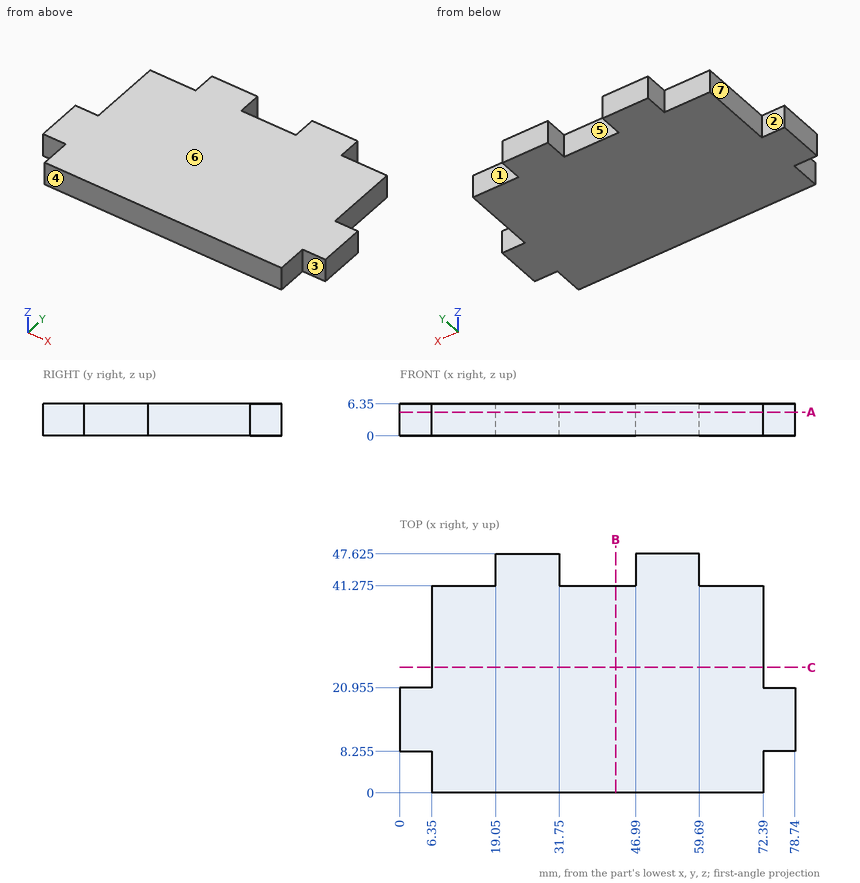
Here's the drawing with two shaded views (mm, measured from the low corner). I have some questions. A direction names the side the tool comes from. Coordinates: 2 decimals unless noted, no trailing zeros. Write each loop counter-clockwise with the first axis right and the second up, starting at its lowest first coordinate (ties: lowest second). Pieces come first, ordered by that corner, then holes.
Item 1: If I drill on line 1 (X direction, y = 43, z = 1.75); line 2 (X direction, y = 36, z = 6); line 3 (Y direction, x = 15, z = 5) (3 decimals), over which ranges is the centre line in solid material (lowest first)?
Item 2: I want a section at C-C on y = 25. Write out the boundary of the cut face in (x, z).
Item 3: I want a section at B-B on x = 43. Write out the boundary of the cut face in (y, z) (3 decimals).
Item 4: Will these pins go through, and if not, where does the flat tip stop? pin 1 (3 mm diameter, centred on x = 76, z = 2, fed in from +Y) (3 decimals); pin 2 (1.9 mm diameter, centred on x = 3.5, z = 3, fed in from -Y) (3 decimals); pin 3 (3 mm diameter, centred on x = 68.5, z = 3, fed in from +Y) (3 decimals).
Item 5: If we mould it in two halves opening along X, with no side actions, what happens to the marked faces 5, 6 and 7? For each: +X half, -X half, draft (parallel to the pull), parting line (faces both ways), or undercut.
Item 6: On a 3-axis mill with a long thin cutter (end or side, diameter ignored), from which of +Z, -Z, +X, -X, +Y, -Y can I reach the whole of each face in a straight line? I mean the marked faces 1, 2, 3 and 4. Say none if no direction works.
Item 7: I want a section at A-A on z = 4.75. Write out the boundary of the cut face in (x, y) (3 decimals).
Findings below:
1. line 1: x = 19.05 to 31.75, 46.99 to 59.69
1. line 2: x = 6.35 to 72.39
1. line 3: y = 0 to 41.275
2. outline: (6.35, 0) - (72.39, 0) - (72.39, 6.35) - (6.35, 6.35) - close
3. outline: (0, 0) - (41.275, 0) - (41.275, 6.35) - (0, 6.35) - close
4. pin 1: stops at y = 20.955
4. pin 2: stops at y = 8.255
4. pin 3: stops at y = 41.275
5. face 5: undercut
5. face 6: draft
5. face 7: -X half
6. face 1: +Z, -Z, +X, +Y
6. face 2: +Z, -Z, -X, +Y
6. face 3: +Z, -Z, +X, -Y
6. face 4: +Z, -Z, +X, -X, -Y
7. outline: (0, 8.255) - (6.35, 8.255) - (6.35, 0) - (72.39, 0) - (72.39, 8.255) - (78.74, 8.255) - (78.74, 20.955) - (72.39, 20.955) - (72.39, 41.275) - (59.69, 41.275) - (59.69, 47.625) - (46.99, 47.625) - (46.99, 41.275) - (31.75, 41.275) - (31.75, 47.625) - (19.05, 47.625) - (19.05, 41.275) - (6.35, 41.275) - (6.35, 20.955) - (0, 20.955) - close
